Geometry: see drawing. Coordinates: mm, zero at the bounding-box minimum. A direction names the side the tool comes from. Round coordinates to 2 decimals unless told otherwise and drop trailing zeros. Write each loop counter-clockwise with the first axis right and the second up, starting at its lowest first coordinate (ties: lowest second). Pieces come first, ordered by that corner, then holes.
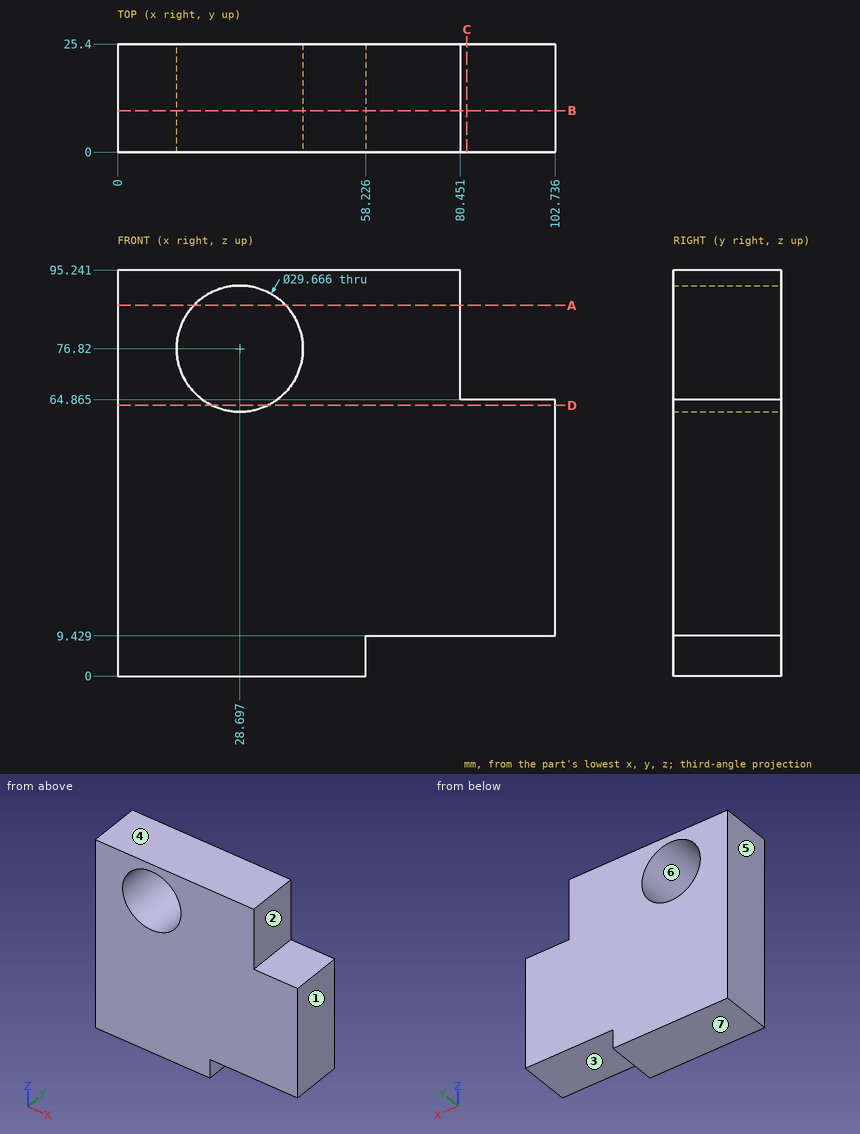
Q1. Section query C-C, the plane x = 82. Output: boundary loops of the cut face in (y, z) (1 decimal), and give its area (3 significant figures).
Q2. Section query B-B, the plane y = 9.75. Output: boundary loops of the cut face in (x, z) (1 decimal), and give its area (3 significant figures).
Q3. Line query: line 1 (X direction, y = 2.75, z = 77.5) (1 decimal); line 2 (Z direction, x = 28, y = 19); line 3 (Z direction, x = 87.5, y = 9) (1 decimal). Output: solid intervals per line, ascending.
Q4. Section query A-A, the plane z = 87. Output: boundary loops of the cut face in (x, y) (1 decimal).
Q5. Mould query, pull axis Z, two halves, no side actions, for the marked faces 4, 5, 6 and 7. Classes: pulls with the +Z half, pulls with the -Z half, needs draft (parallel to the pull), parting line crosses it, or undercut.
Q6. Set-up query: the marked faces 1, 2 and 3. Return all of +Z, -Z, +X, -X, +Y, -Y with unobstructed straight access to the full face (end or side cutting, diameter ignored); none if empty.
Q7. Section query D-D, the plane z = 63.5. Output: boundary loops of the cut face in (x, y) (1 decimal).
Filled in:
1. outline: (0, 9.4) - (25.4, 9.4) - (25.4, 64.9) - (0, 64.9) - close
1. area: 1,410 mm2
2. outline: (0, 0) - (58.2, 0) - (58.2, 9.4) - (102.7, 9.4) - (102.7, 64.9) - (80.5, 64.9) - (80.5, 95.2) - (0, 95.2) - close; hole circle Ø29.7 at (28.7, 76.8)
2. area: 8,000 mm2
3. line 1: x = 0 to 13.9, 43.5 to 80.5
3. line 2: z = 0 to 62, 91.64 to 95.24
3. line 3: z = 9.4 to 64.9
4. outline: (0, 0) - (17.9, 0) - (17.9, 25.4) - (0, 25.4) - close; (39.5, 0) - (80.5, 0) - (80.5, 25.4) - (39.5, 25.4) - close
5. face 4: pulls with the +Z half
5. face 5: needs draft
5. face 6: undercut
5. face 7: pulls with the -Z half
6. face 1: +Z, -Z, +X, +Y, -Y
6. face 2: +Z, +X, +Y, -Y
6. face 3: -Z, +X, +Y, -Y
7. outline: (0, 0) - (22.2, 0) - (22.2, 25.4) - (0, 25.4) - close; (35.2, 0) - (102.7, 0) - (102.7, 25.4) - (35.2, 25.4) - close
